Here's how the part is built. I have some questions about the finished solid (model axes, mm). Coordinates: 2 decimals unless noted, no trailing zeros. Loops run counter-clockwise (first coordinate to the right, second up) from the corner with the lowest first, then second, coordinate; pieces in that order, holes last.
Autodesk Inventor part; units mm, degrees
ref_plane "YZ Plane" through (0, 0, 0) normal (1, 0, 0) x (0, 1, 0)
ref_plane "XZ Plane" through (0, 0, 0) normal (0, 1, 0) x (-1, 0, 0)
ref_plane "XY Plane" through (0, 0, 0) normal (0, 0, 1) x (1, 0, 0)
sketch "スケッチ1" plane through (0, 0, 0) normal (0, 1, 0) x (-1, 0, 0)
  circle A0 centre (55.3, 11.85) radius 2.1
  circle A1 centre (31.1, 14.7) radius 2.1
  circle A2 centre (6.9, 11.85) radius 2.1
  line L0 (62.1, 5.5) -> (0.1, 5.5)
  line L1 (2.1, 20) -> (60.1, 20)
  line L2 (2.1, 20) -> (18.1, 20)
  line L3 (-0.9, 6.5) -> (-0.9, 17)
  line L4 (63.1, 17) -> (63.1, 6.5)
  line L5 (63.1, 17) -> (60.1, 20)
  line L6 (-0.9, 17) -> (2.1, 20)
  line L7 (63.1, 6.5) -> (62.1, 5.5)
  line L8 (0.1, 5.5) -> (-0.9, 6.5)
  point P0 (0, 0)
  point P1 (-0.9, 5.5)
  point P2 (-0.9, 20)
  point P3 (63.1, 20)
  point P4 (63.1, 5.5)
  dimension "d0" = 64
  dimension "d2" = 14.5
  dimension "d3" = 4.2
  dimension "d4" = 4.2
  dimension "d5" = 4.2
  dimension "d8" = 3
  dimension "d9" = 3
  dimension "d10" = 3
  dimension "d11" = 3
  dimension "d12" = 1
  dimension "d13" = 1
  dimension "d14" = 1
  dimension "d15" = 1
extrude "押し出し1" add sketch "スケッチ1" along normal blind 3
equation "\"d4\" = d3"
equation "\"d5\" = d4"
properties part number "stopperver2_1"
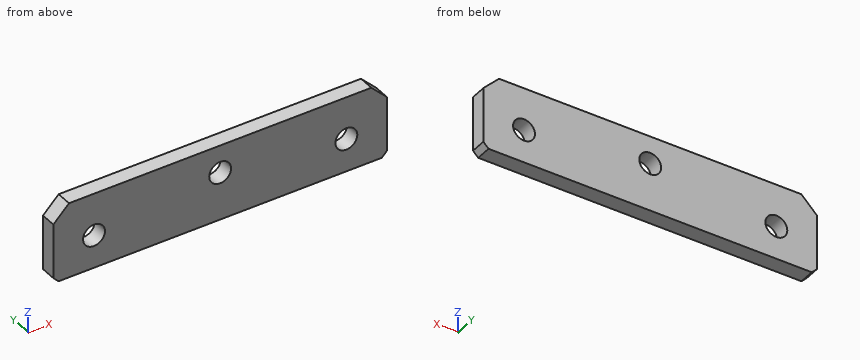
Q1. Will this pin go through, and if not, where does the flat tip stop? P1, Ø3.5, axis at x = -55.3, z = 11.85, coming from the +Y side.
Q2. Suppose I cut it at A-A on x = -6.9. Write out the boundary of the cut face in (y, z), and give its area (3 significant figures).
Q3. Suppose I cut it at C-C on y = 2.4. Write out the boundary of the cut face in (x, z).
Q4. Suppose I cut it at B-B on z = 11.85. Write out the boundary of the cut face in (x, y), and give its area (3 significant figures).
Q5. Please list where these lines run through material, in increasing order: probe 1 along Z at (x, y) = (-55.3, 0.8); probe 2 along X at (y, z) = (1.4, 10); probe 3 along X at (y, z) = (2.05, 10.75).
Q6. Suppose I cut it at D-D on z = 16.25. Write out the boundary of the cut face in (x, y).
Check values:
1. P1: passes through
2. outline: (0, 5.5) - (3, 5.5) - (3, 9.75) - (0, 9.75) - close; (0, 13.95) - (3, 13.95) - (3, 20) - (0, 20) - close
2. area: 30.9 mm2
3. outline: (-63.1, 6.5) - (-62.1, 5.5) - (-0.1, 5.5) - (0.9, 6.5) - (0.9, 17) - (-2.1, 20) - (-60.1, 20) - (-63.1, 17) - close; hole circle Ø4.2 at (-55.3, 11.85); hole circle Ø4.2 at (-31.1, 14.7); hole circle Ø4.2 at (-6.9, 11.85)
4. outline: (-63.1, 0) - (-57.4, 0) - (-57.4, 3) - (-63.1, 3) - close; (-53.2, 0) - (-9, 0) - (-9, 3) - (-53.2, 3) - close; (-4.8, 0) - (0.9, 0) - (0.9, 3) - (-4.8, 3) - close
4. area: 167 mm2
5. probe 1: z = 5.5 to 9.75, 13.95 to 20
5. probe 2: x = -63.1 to -56.29, -54.31 to -7.89, -5.91 to 0.9
5. probe 3: x = -63.1 to -57.09, -53.51 to -8.69, -5.11 to 0.9
6. outline: (-63.1, 0) - (-32.52, 0) - (-32.52, 3) - (-63.1, 3) - close; (-29.68, 0) - (0.9, 0) - (0.9, 3) - (-29.68, 3) - close
